Job drawing, mm, ordinate dimensions from the low corner. One solid piece. Round coordinates to 2 decimals unless told otherwise and drop trailing zeros. Loops run counter-clockwise (first coordinate to the right, second up) from the corner with the lowest first, then second, coordinate; pieces in that order, holes last. Notation, with made-up numbers: M -26.5,35 L -4.5,35 A35 ccw -4.5,72 Z; hole C 32.5,44.25 d9. An arc over 180 degrees is marked long. Write each question's results on one line, items separated by ' | '. Start each with the question number.
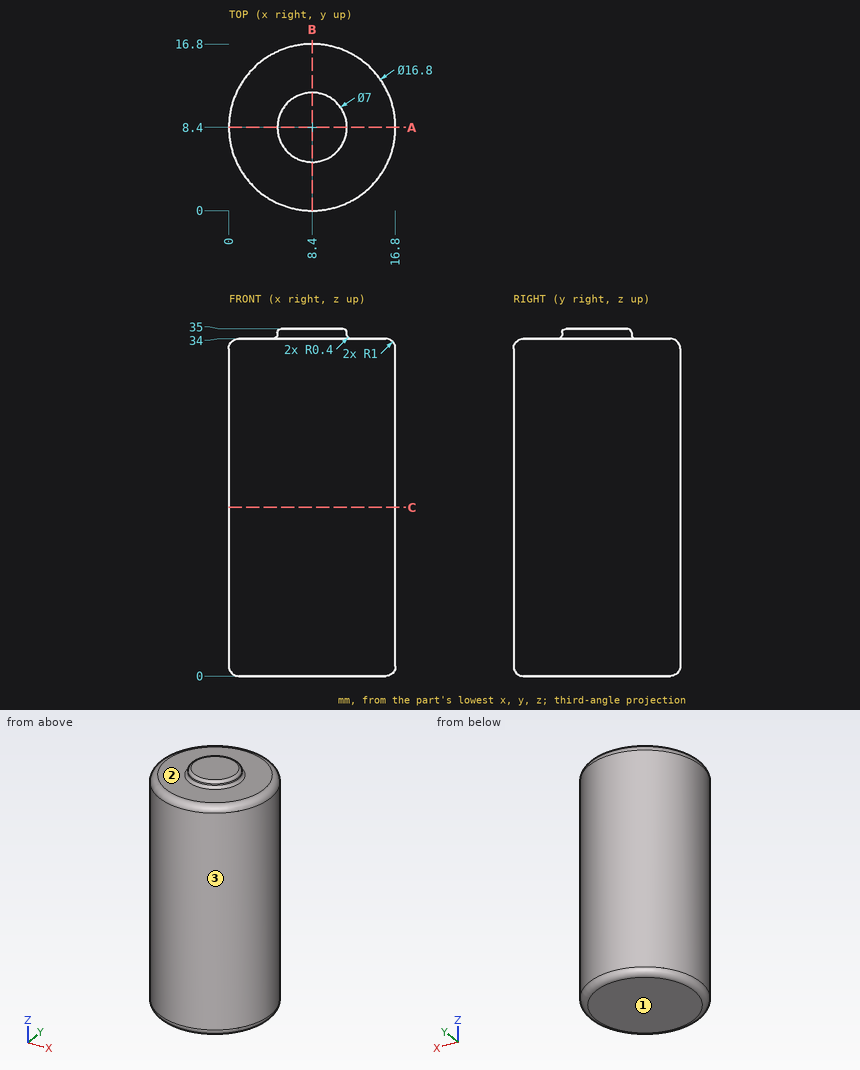
Item 1: Drop flat-ended pins along their axis: pin 1 (10 mm diameter, centred on y = 11, z = 12, fed in from -X); pin 2 (4 mm diameter, centred on y = 12.5, z = 28.5, fed in from -X); pin 3 (1 mm diameter, centred on x = 13, y = 2.5, fed in from +Z); pin 4 (6 mm diameter, centred on y = 14, z = 23.5, fed in from +X). Give the stop position or say it passes through.
Item 2: Drill centre lines: line 1 along Z through (x, y) = (1.5, 10.75); line 2 along Z through (x, y) = (5.25, 8); line 3 along X through (y, z) = (8.75, 31.5). Where is each one in solid material? Low to high. Write a range as [from, to].
Item 3: Mould opens along Z. For the marked faces 1, 2 and 3 say: released by +Z, released by -Z, zero draft, split by the parting line, or undercut.
Item 4: Saw through at A-A, the plane y = 8.4. Give the cut face in (x, z).
Item 5: Saw through at C-C, the plane z = 17. Give the cut face in (x, y), then the cut area to 3 significant figures.
Working result:
1) pin 1: stops at x = 0 | pin 2: stops at x = 0.27 | pin 3: stops at z = 34 | pin 4: stops at x = 16.39
2) line 1: z = [0, 34] | line 2: z = [0, 34.99] | line 3: x = [0.01, 16.79]
3) face 1: released by -Z | face 2: released by +Z | face 3: zero draft
4) outline: M 0,1 A1 ccw 1,0 L 15.8,0 A1 ccw 16.8,1 L 16.8,33 A1 ccw 15.8,34 L 12.3,34 A0.4 cw 11.9,34.4 L 11.9,34.6 A0.4 ccw 11.5,35 L 5.3,35 A0.4 ccw 4.9,34.6 L 4.9,34.4 A0.4 cw 4.5,34 L 1,34 A1 ccw 0,33 Z
5) outline: C 8.4,8.4 d16.8 | area: 222 mm²
